Geometry check sheet. Reference: the model listing, model coordinates, mm. A direction names the side the tool comes from. Give positions to 0.01 mm unless a question says otherwise; leave off trailing zeros. Order: outer loops, then holes, each group sorted by start corner. A loop starts at its lowest first (then second) coordinate and runs counter-clockwise, first axis right, second up. Notation, with made-up numbers: M 44.25,-23 L 99.25,-23 A30 cw 99.25,12 Z; hole C -1.5,-10 d1. An arc over 180 degrees is marked long. Answer as CSV lines item,"result". Start each with the question number.
```python
from build123d import *

# Parameters (mm, degrees)
SCHIZZO1_W                    = 29.96
SCHIZZO1_H                    = 29.94
ESTRUSIONE_ESTRUSIONE1_DEPTH  = 5.1
TAGLIO_ESTRUSIONE1_DEPTH      = 5.1
SCHIZZO3_R                    = 1.5
TAGLIO_ESTRUSIONE2_DEPTH      = 22.783280286
FORO_FILETTATO_M3X0_5_1_D     = 2.5
FORO_FILETTATO_M3X0_5_2_D     = 2.5
FORO_FILETTATO_M3X0_5_2_DEPTH = 10
FORO_FILETTATO_M3X0_5_2_TIP   = 0.751075774


with BuildPart() as part:
    # Schizzo1 → Estrusione-Estrusione1 (new body)
    with BuildSketch(Plane(origin=(0, 0, 0), x_dir=(1, 0, 0), z_dir=(0, 1, 0))):
        Rectangle(SCHIZZO1_W, SCHIZZO1_H)
    extrude(amount=-ESTRUSIONE_ESTRUSIONE1_DEPTH)

    # Schizzo2 → Taglio-Estrusione1 (cut)
    with BuildSketch(Plane(origin=(0, 0, 0), x_dir=(1, 0, 0), z_dir=(0, 1, 0))):
        Polygon((-4.98, -8.17), (-8.90598183, -14.97), (8.90598183, -14.97), (4.98, -8.17), align=None)
        with BuildLine():
            ThreePointArc((14.98, 8), (12.065, 0), (14.98, -8))
            Line((14.98, -8), (14.98, 8))
        make_face()
        with BuildLine():
            Line((9.38, 14.97), (-9.38, 14.97))
            Line((-9.38, 14.97), (-7.05655311, 10.945671938))
            ThreePointArc((-7.05655311, 10.945671938), (-5.469571784, 10.139327056), (-4.09, 11.264264161))
            ThreePointArc((-4.09, 11.264264161), (0, 14.25), (4.09, 11.264264161))
            ThreePointArc((4.09, 11.264264161), (5.469571784, 10.139327056), (7.05655311, 10.945671938))
            Line((7.05655311, 10.945671938), (9.38, 14.97))
        make_face()
        with BuildLine():
            Line((-14.98, 8), (-14.98, -8))
            ThreePointArc((-14.98, -8), (-12.065, 0), (-14.98, 8))
        make_face()
    extrude(amount=-TAGLIO_ESTRUSIONE1_DEPTH, mode=Mode.SUBTRACT)

    # Schizzo3 → Taglio-Estrusione2 (cut, through all)
    with BuildSketch(Plane(origin=(0, 0, 0), x_dir=(1, 0, 0), z_dir=(0, 1, 0))):
        with Locations(Location((0, 10.34, 0), (0, 0, 270))):
            Circle(SCHIZZO3_R)
        with Locations(Location((0, 2.58, 0), (0, 0, 270))):
            Circle(SCHIZZO3_R)
    extrude(amount=-TAGLIO_ESTRUSIONE2_DEPTH, mode=Mode.SUBTRACT)

    # Foro filettato M3x0.5-1 (through all)
    with Locations(Plane(origin=(0, 0, 0), x_dir=(1, 0, 0), z_dir=(0, 1, 0))):
        with Locations((0, -3.17)):
            Hole(FORO_FILETTATO_M3X0_5_1_D / 2)

    # Foro filettato M3x0.5-2
    with Locations(Plane(origin=(16.95, 0, 0), x_dir=(0, 0, -1), z_dir=(1, 0, 0))):
        with Locations((-12.23, -2.72), (11.87, -2.72)):
            Hole(FORO_FILETTATO_M3X0_5_2_D / 2, depth=FORO_FILETTATO_M3X0_5_2_DEPTH)
            with Locations((0, 0, -(FORO_FILETTATO_M3X0_5_2_DEPTH + FORO_FILETTATO_M3X0_5_2_TIP / 2))):  # 118° drill point
                Cone(0, FORO_FILETTATO_M3X0_5_2_D / 2, FORO_FILETTATO_M3X0_5_2_TIP, mode=Mode.SUBTRACT)


solid = part.part
```
Item 1: Draft check along Z on faces 1 (the face through (14.98, -2.5, 10.8)), 2 (the face through (0.07, -2.51, -4.08)), 3 (the face through (8.46, -2.51, -13.38)). Enter one of: pulls with the +Z half, pulls with the -Z half, needs draft (parallel to the pull), parting line crosses it, or undercut.
Item 2: Section check C-C on x = -0.5. Record the boundary of the cut face in (y, z), then the cut area to 3 significant figures.
Item 3: Section check A-A on y = -2.72. Give the number of separate pieces and of enclosed holes in the cut face, then the cut area to 3 significant figures.
Item 4: Section check D-D on z = -2.58. Record the boundary of the cut face in (x, y), then the cut area to 3 significant figures.
Item 5: Scan lines: line 1 along Z through (x, y) = (10.5, -2.72); line 2 along Z through (x, y) = (0.75, -1.7); line 3 along X through (y, z) = (-4.65, -2.5). Record each from-to range of solid material in increasing order.
Item 6: Section check B-B on z = 12.23. Record the boundary of the cut face in (x, y).
Item 7: Depth check by flat-ended pin: pin 1 Ø2.5 at (x, z) = (0, -10.34) entering from +Y; pin 2 Ø3 at (y, z) = (-4, 6) entering from -X; pin 3 Ø1.5 at (x, y) = (-1.5, -3) entering from +Z; pin 4 Ø1.5 at (x, y) = (-8.5, -3.5) entering from -Z. Enter the tip coordinate at first touch or a pass-through.
Item 8: Access from +Z, -Z, +X, -X, +Y, -Y to the whole of each face (thin tool, end or side, straight path). Record for faces 4 (the face through (0, -3, 8.17)), 5 (the face through (-8.235, -2.514, -12.986)), 6 (the face through (12, -3, 14.97)).
Numbers:
1,face 1,"needs draft"
1,face 2,"undercut"
1,face 3,"pulls with the -Z half"
2,outline,"M -5.1,-14.22 L 0,-14.22 L 0,-11.75 L -5.1,-11.75 Z; M -5.1,-8.93 L 0,-8.93 L 0,-3.99 L -5.1,-3.99 Z; M -5.1,-1.17 L 0,-1.17 L 0,2.02 L -5.1,2.02 Z; M -5.1,4.32 L 0,4.32 L 0,8.17 L -5.1,8.17 Z"
2,area,"73.7 mm2"
3,separate pieces,"3"
3,enclosed holes,"3"
3,area,"633 mm2"
4,outline,"M -12.34,-5.1 L -1.5,-5.1 L -1.5,0 L -12.34,0 Z; M 1.5,-5.1 L 12.34,-5.1 L 12.34,0 L 1.5,0 Z"
4,area,"111 mm2"
5,line 1,"-14.97 to -13.12, -10.62 to 10.98, 13.48 to 14.97"
5,line 2,"-14.18 to -11.64, -9.04 to -3.88, -1.28 to 2.17, 4.17 to 8.17"
5,line 3,"-12.32 to -1.5, 1.5 to 12.32"
6,outline,"M -14.98,-5.1 L -7.32,-5.1 L -7.32,0 L -14.98,0 Z; M 7.32,-5.1 L 14.98,-5.1 L 14.98,-3.97 L 7.32,-3.97 Z; M 7.32,-1.47 L 14.98,-1.47 L 14.98,0 L 7.32,0 Z"
7,pin 1,"through"
7,pin 2,"x = -14.58"
7,pin 3,"z = 8.17"
7,pin 4,"z = -14.74"
8,face 4,"+Z, +Y, -Y"
8,face 5,"-Z, +Y, -Y"
8,face 6,"+Z, +X, -X, +Y, -Y"
